For this review, take the finished solid that the model builds, in its own axes (mm). Round coordinates to 2 decimals unless told otherwise and drop trailing zeros. Write each loop counter-clockwise with the first axis right and the second up, starting at its lowest first coordinate (ties: lowest second). Pieces come first, ordered by that corner, then holes. Notation, with made-up numbers: (84.25, 24.25) - (98.25, 24.25) arc R21 cw to (98.25, 56.25) - close; hole circle Ø1 at (-31, 4.25). An arc over 180 degrees is marked (long way). Answer in a Markdown table with one row per item. Add a question column.
Autodesk Inventor part; units mm, degrees
ref_plane "YZ Plane" through (0, 0, 0) normal (1, 0, 0) x (0, 1, 0)
ref_plane "XZ Plane" through (0, 0, 0) normal (0, 1, 0) x (-1, 0, 0)
ref_plane "XY Plane" through (0, 0, 0) normal (0, 0, 1) x (1, 0, 0)
sketch "Sketch1" plane through (0, 0, 0) normal (0, 0, 1) x (1, 0, 0)
  line L0 (0, 0) -> (0, 4438.8737)
  line L1 (0, 4438.8737) -> (100, 4438.8737)
  line L2 (100, 4438.8737) -> (200, 0)
  line L3 (200, 0) -> (0, 0)
  circle A0 centre (0, 0) radius 30
  line L4 (0, 1479.6246) -> (166.6667, 1479.6246)
  line L5 (0, 2959.2492) -> (133.3333, 2959.2492)
  circle A1 centre (0, 1479.6246) radius 30
  circle A2 centre (0, 2959.2492) radius 30
  line L6 (190.4255, 425) -> (120.4255, 425)
  line L7 (120.4255, 425) -> (120.4255, 430)
  line L8 (120.4255, 430) -> (190.4255, 430)
  line L9 (190.4255, 430) -> (190.4255, 425)
  line L10 (109.1642, 929.8732) -> (179.1642, 929.8732)
  line L11 (179.1642, 924.8732) -> (109.1642, 924.8732)
  line L12 (109.1642, 924.8732) -> (109.1642, 929.8732)
  line L13 (179.1642, 929.8732) -> (179.1642, 924.8732)
  line L14 (97.903, 1429.7463) -> (167.903, 1429.7463)
  line L15 (167.903, 1424.7463) -> (97.903, 1424.7463)
  line L16 (97.903, 1424.7463) -> (97.903, 1429.7463)
  line L17 (167.903, 1429.7463) -> (167.903, 1424.7463)
  line L18 (86.6417, 1929.6195) -> (156.6417, 1929.6195)
  line L19 (156.6417, 1924.6195) -> (86.6417, 1924.6195)
  line L20 (86.6417, 1924.6195) -> (86.6417, 1929.6195)
  line L21 (156.6417, 1929.6195) -> (156.6417, 1924.6195)
  line L22 (75.3805, 2429.4927) -> (145.3805, 2429.4927)
  line L23 (145.3805, 2424.4927) -> (75.3805, 2424.4927)
  line L24 (75.3805, 2424.4927) -> (75.3805, 2429.4927)
  line L25 (145.3805, 2429.4927) -> (145.3805, 2424.4927)
  line L26 (64.1192, 2929.3658) -> (134.1192, 2929.3658)
  line L27 (134.1192, 2924.3658) -> (64.1192, 2924.3658)
  line L28 (64.1192, 2924.3658) -> (64.1192, 2929.3658)
  line L29 (134.1192, 2929.3658) -> (134.1192, 2924.3658)
  line L30 (52.8579, 3429.239) -> (122.8579, 3429.239)
  line L31 (122.8579, 3424.239) -> (52.8579, 3424.239)
  line L32 (52.8579, 3424.239) -> (52.8579, 3429.239)
  line L33 (122.8579, 3429.239) -> (122.8579, 3424.239)
  line L34 (41.5967, 3929.1122) -> (111.5967, 3929.1122)
  line L35 (111.5967, 3924.1122) -> (41.5967, 3924.1122)
  line L36 (41.5967, 3924.1122) -> (41.5967, 3929.1122)
  line L37 (111.5967, 3929.1122) -> (111.5967, 3924.1122)
  line L38 (0, 1629.6246) -> (163.2874, 1629.6246)
  line L39 (0, 3039.2492) -> (131.5311, 3039.2492)
  point P0 (30, 2959.2492)
  point P1 (0, 2929.2492)
  point P2 (0, 1509.6246)
  point P3 (0, 1449.6246)
  point P4 (0, 30)
  point P5 (30, 0)
  point P6 (190.3129, 430)
  point P7 (179.0516, 929.8732)
  point P8 (167.7903, 1429.7463)
  point P9 (30, 1479.6246)
  dimension "d65" = 100
  dimension "d67" = 200
  dimension "d68" = 60
  dimension "d69" = 1480
  dimension "d70" = 1480
  dimension "d71" = 1480
  dimension "d72" = 5
  dimension "d73" = 70
  dimension "d74" = 430
  dimension "d77" = 500
  dimension "d82" = 80
  dimension "d83" = 150
extrude "Plate3" add sketch "Sketch1" along normal blind 4 contours L38 L2 L4 A1 L0 | L4 L2 L14 L16 L15 L10 L12 L11 L8 L7 L6 L3 A0 L0 A1
chamfer "Corner Chamfer2" distance 3 angle 45 6 edges at (190.3129, 430, 2) (190.4255, 425, 2) (179.1642, 924.8732, 2) (179.0516, 929.8732, 2) (167.903, 1424.7463, 2) (167.7903, 1429.7463, 2)
equation "\"BendRadius\" = Thickness"
equation "\"BendReliefWidth\" = Thickness"
equation "\"BendReliefDepth\" = 0.5 * Thickness"
equation "\"CornerReliefSize\" = 4 * Thickness"
equation "\"MinimumRemnant\" = 2 * Thickness"
equation "\"TransitionRadius\" = BendRadius"
equation "\"JacobiRadiusSize\" = BendRadius"
equation "\"GapSize\" = Thickness"
properties part number "GBK 3101 Center main rib" material "Steel"
Q1. Add section B-B on y = 981.5. State the section outline as (x, z) points.
Q2. Insertion check: pin 1 Ø2 at (x, z) = (162, 1) entering from -Y; pin 2 Ø2 at (y, z) = (1427.5, 2.5) entering from +X; pin 3 Ø2 at (y, z) = (426.5, 1.5) entering from +X. Each pin has a flat end and moves straight along its axis. Give the tip position at first contact, or say it passes through.
Q3. Add section C-C on y = 606. State the section outline as (x, z) points, then the cut area to 3 significant figures.
Q4. Add section A-A on z = 1.15. State the section outline as (x, y) points.
Q5. To check wall thickness, follow probe 1 along Y at (x, z) = (145.5, 1.65); probe 2 along Y at (x, z) = (112.5, 3.7); probe 3 along Y at (x, z) = (105.5, 1.65). State the ranges of each line that lie inside material, in increasing order.
Q6. Draft analysis for pull direction Y (two halves, no side actions). For faces 1 (the face through (29.993, 1480.284, 1.972)), 2 (the face through (99, 826, 0)), 3 (the face through (20.979, 21.445, 1.972)), state which applies: released by +Y, released by -Y, zero draft, split by the parting line, or undercut.
Answer sheet:
| question | item | result |
|---|---|---|
| 1 | outline | (0, 0) - (177.89, 0) - (177.89, 4) - (0, 4) - close |
| 2 | pin 1 | stops at y = 0 |
| 2 | pin 2 | stops at x = 97.9 |
| 2 | pin 3 | stops at x = 120.43 |
| 3 | outline | (0, 0) - (186.35, 0) - (186.35, 4) - (0, 4) - close |
| 3 | area | 745 mm² |
| 4 | outline | (0, 30) arc R30 cw to (30, 0) - (200, 0) - (190.49, 422) - (187.43, 425) - (120.43, 425) - (120.43, 430) - (187.31, 430) - (190.25, 433) - (179.23, 921.87) - (176.16, 924.87) - (109.16, 924.87) - (109.16, 929.87) - (176.05, 929.87) - (178.98, 932.87) - (167.97, 1421.75) - (164.9, 1424.75) - (97.9, 1424.75) - (97.9, 1429.75) - (164.79, 1429.75) - (167.72, 1432.75) - (163.29, 1629.62) - (0, 1629.62) - (0, 1509.62) arc R30 cw to (0, 1449.62) - close |
| 5 | probe 1 | y = 0 to 425, 430 to 924.87, 929.87 to 1424.75, 1429.75 to 1629.62 |
| 5 | probe 2 | y = 0 to 924.87, 929.87 to 1424.75, 1429.75 to 1629.62 |
| 5 | probe 3 | y = 0 to 1424.75, 1429.75 to 1629.62 |
| 6 | face 1 | undercut |
| 6 | face 2 | zero draft |
| 6 | face 3 | released by -Y |
